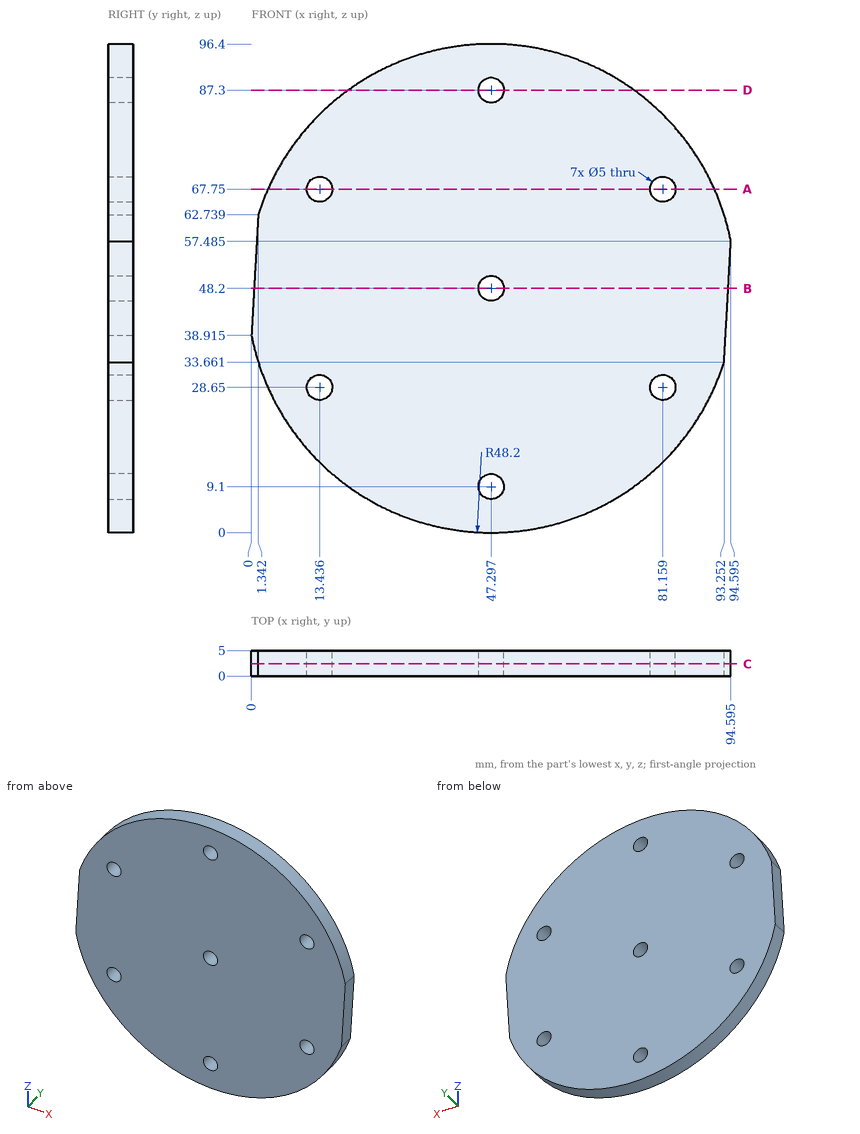
Input: dimensioned drawing with shaded views. Units: mm. Origin: part minimum x, y, z. Coordinates: 2 decimals unless noted, no trailing zeros. Write each loop counter-clockwise with the first axis right and the second up, starting at its lowest first coordinate (ties: lowest second). Pieces come first, ordered by that corner, then holes. Notation, with made-up numbers: M -4,49.25 L 3,49.25 A26 cw 3,64.25 Z; hole C -39,-11 d2. An arc over 180 degrees is marked long. Answer as a JSON object with one key per item and string values. Group by question number.
(1) Contact query for flat-ended pins moving along their axis: P1, Ø3, axis at y = 3.5, z = 33.5, coming from the -X side; P2, Ø3, axis at x = 47.3, z = 48.2, coming from the -Y side; P3, Ø2, axis at y = 1.5, z = 10, coming from the -X side; P4, Ø2, axis at x = 68.5, y = 1.5, coming from the -Z side. Output: stop coordinate, or through.
(2) Section A-A on z = 67.75. Output: boundary loops of the cut face in (x, y) (1 decimal).
(3) Section C-C on y = 2.4. Give the number of separate pieces and of enclosed holes in the cut face, plus the area to 3 significant figures.
(4) Section D-D on z = 87.3. Output: boundary loops of the cut face in (x, y).
(5) Ray query, line 1 along Z through (x, y) = (49, 2.5); line 2 along X through (y, z) = (3.1, 28.65) (1 decimal). Return the intervals inside material, ascending. Write a range as [from, to].
(6) Section B-B on z = 48.2. Output: boundary loops of the cut face in (x, y).
Result set:
{
 "1": {"P1": "stops at x = 0.94", "P2": "passes through", "P3": "stops at x = 16.65", "P4": "stops at z = 4.44"},
 "2": {"outline": "M 3.2,0 L 10.9,0 L 10.9,5 L 3.2,5 Z; M 15.9,0 L 78.7,0 L 78.7,5 L 15.9,5 Z; M 83.7,0 L 91.4,0 L 91.4,5 L 83.7,5 Z"},
 "3": {"separate pieces": "1", "enclosed holes": "7", "area": "7,110 mm2"},
 "4": {"outline": "M 19.11,0 L 44.8,0 L 44.8,5 L 19.11,5 Z; M 49.8,0 L 75.48,0 L 75.48,5 L 49.8,5 Z"},
 "5": {"line 1": "z = [0.03, 7.27], [10.93, 46.37], [50.03, 85.47], [89.13, 96.37]", "line 2": "x = [3.2, 10.9], [15.9, 78.7], [83.7, 91.4]"},
 "6": {"outline": "M 0.52,0 L 44.8,0 L 44.8,5 L 0.52,5 Z; M 49.8,0 L 94.07,0 L 94.07,5 L 49.8,5 Z"}
}
